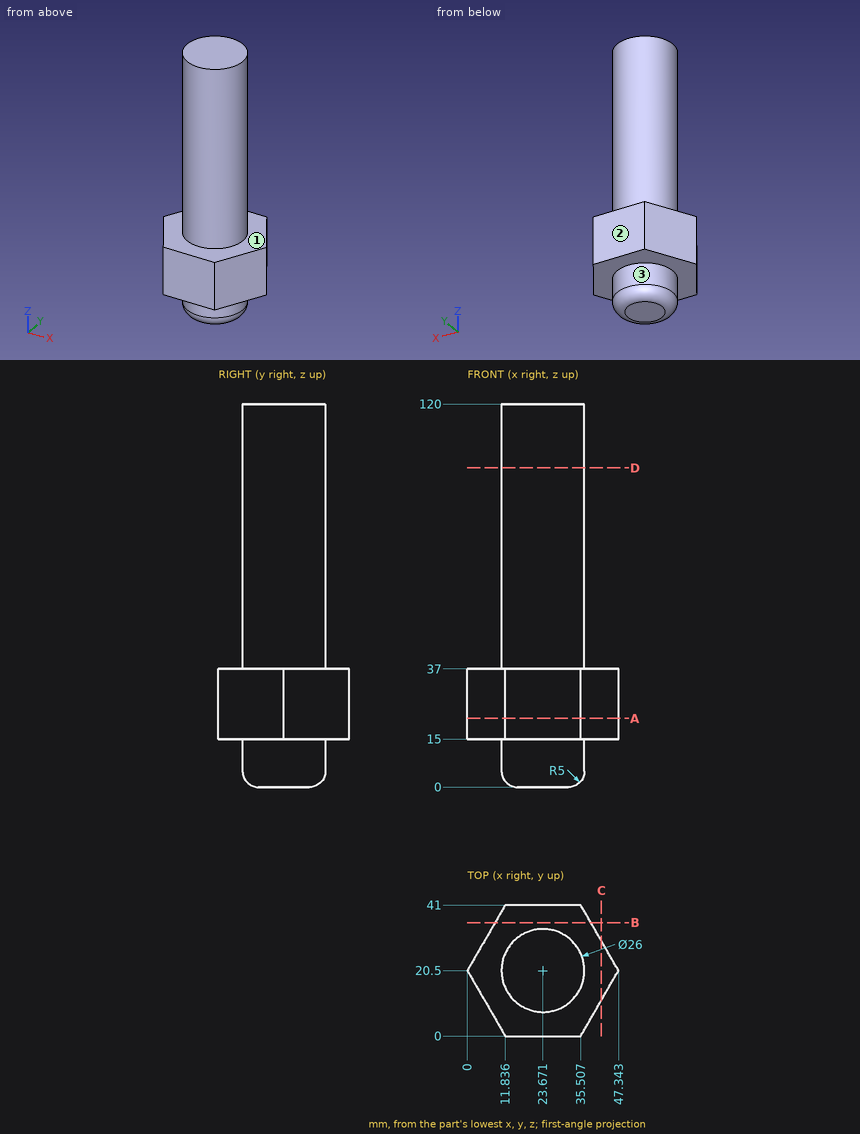
Part print with two shaded views. Sizes in mm from the minimum x, y, z corner. A direction names the side the tool comes from. Coordinates: 2 decimals unless noted, no trailing zeros. Order: outer loops, then holes, each group sorted by start corner. A loop starts at its lowest first (then second) coordinate and runs counter-clockwise, first axis right, second up.
(1) Saw through at D-D, the plane z = 100. Write the cut outline in (x, y), and give its area (3 significant figures).
Solution:
outline: circle Ø26 at (23.67, 20.5)
area: 531 mm2
(2) Drill centre lines: L1, parallel to Z at x = 43, y = 24; L2, parallel to Y at x = 34, z = 58 (1 decimal); L3, parallel to Y at x = 22, z = 97.5. Where is each one in solid material? Low to high.
Solution:
L1: z = 15 to 37
L2: y = 12.6 to 28.4
L3: y = 7.61 to 33.39
(3) Saw through at B-B, the plane y = 35.5. Write the cut outline in (x, z).
Solution:
outline: (8.66, 15) - (38.68, 15) - (38.68, 37) - (8.66, 37) - close
(4) Which spindle directions (+Z, -Z, +X, -X, +Y, -Y) get a long thin tool onto all of the face, cutting with end or side? Do the marked faces 1, 2 and 3. Say none if no direction does.
Solution:
face 1: +Z
face 2: +Z, -Z, +X, -X, +Y
face 3: -Z
(5) Saw through at C-C, the plane x = 42. Write the cut outline in (y, z).
Solution:
outline: (11.25, 15) - (29.75, 15) - (29.75, 37) - (11.25, 37) - close
(6) Saw through at A-A, the plane z = 21.5. Write the cut outline in (x, y) (1 decimal), and give its area (3 significant figures).
Solution:
outline: (0, 20.5) - (11.8, 0) - (35.5, 0) - (47.3, 20.5) - (35.5, 41) - (11.8, 41) - close
area: 1,460 mm2
(7) Pin check, flat tips, straight feed: pin 1 Ø3 at (y, z) = (30.5, 61) entering from +X; pin 2 Ø6 at (x, y) = (9.5, 32.5) entering from -Z; pin 3 Ø1.5 at (x, y) = (14, 9.5) entering from +Z; pin 4 Ø20.5 at (x, y) = (12.5, 26.5) entering from -Z. Stop position of each tip, or through.
Solution:
pin 1: stops at x = 33.51
pin 2: stops at z = 15
pin 3: stops at z = 37
pin 4: stops at z = 0
